Autodesk Inventor part; units mm, degrees
ref_plane "YZ Plane" through (0, 0, 0) normal (1, 0, 0) x (0, 1, 0)
ref_plane "XZ Plane" through (0, 0, 0) normal (0, 1, 0) x (-1, 0, 0)
ref_plane "XY Plane" through (0, 0, 0) normal (0, 0, 1) x (1, 0, 0)
sketch "Sketch1" plane through (0, 0, 0) normal (0, 1, 0) x (-1, 0, 0)
  line L0 (0, 0) -> (50, 0)
  line L1 (50, 0) -> (50, 12.5)
  line L2 (50, 12.5) -> (75, 12.5)
  line L3 (75, 12.5) -> (75, -37.5)
  line L4 (75, -37.5) -> (50, -37.5)
  line L5 (50, -37.5) -> (50, -25)
  line L6 (50, -25) -> (0, -25)
  line L7 (0, -25) -> (0, 0)
  dimension "d0" = 25
  dimension "d1" = 50
  dimension "d2" = 50
  dimension "d3" = 25
extrude "Extrusion1" add sketch "Sketch1" along normal blind 4
sketch "Sketch2" plane through (0, 4, 0) normal (0, 1, 0) x (1, 0, 0)
  circle A0 centre (-15, 12.5) radius 2.75
  circle A1 centre (-35, 12.5) radius 2.75
  circle A2 centre (-62.5, 2.5) radius 2.75
  circle A3 centre (-62.5, 22.5) radius 2.75
  line L0 (-75, -12.5) -> (-50, -12.5)
  line L1 (-62.5, -12.5) -> (-62.5, 37.5) construction
  line L2 (-50, 37.5) -> (-75, 37.5)
  point P0 (0, 0)
  dimension "d6" = 5.5
  dimension "d7" = 5.5
  dimension "d8" = 20
  dimension "d9" = 10
extrude "Extrusion2" cut sketch "Sketch2" against normal through all
fillet "Fillet1" radius 10 2 edges at (-50, 2, 0) (-50, 2, -25)
equation "\"d9\" = 0.5 * d8"
properties part number "Support Extrusion Brace" material "CFRP"
Work out the finished part from the listing and answer in its coordinate system (mm). A direction names the side the tool comes from. Coordinates: 2 decimals unless noted, no trailing zeros. Loops run counter-clockwise (first coordinate to the right, second up) from the corner with the lowest first, then second, coordinate; pieces in that order, holes last. Notation, with made-up numbers: M 86.25,59 L 132.25,59 A12 ccw 132.25,81 Z; hole C 52.25,27 d7. An arc over 180 degrees is marked long. Answer in a Markdown table with one row per item. Add a question column.
1. Find section C-C, the plane x = -62.5. Write down the section's boundary in (y, z).
2. A tool of negligible diameter and unlimited length cuts with its end or side. For faces 1 (the flat face through (-20, 2, 0)), 2 (the flat face through (-20, 2, -25)), 3 (the flat face through (-45, 0, -12)), from which of +Z, -Z, +X, -X, +Y, -Y can it reach the whole face along a straight path? Write none if from no direction.
3. Find section B-B, the plane z = -12.5. Write down the section's boundary in (x, y), then the cut area to 3 significant figures.
4. The mould has two halves that part along Z. Classify faces 4 (the flat face through (-62, 2, 12.5)), 5 (the flat face through (-50, 2, -36)), 6 (the cylindrical face through (-65.247, 2.028, -22.621)): pulls with the +Z half, pulls with the -Z half, needs draft (parallel to the pull), parting line crosses it, or undercut.
5. Flat-ended cylindrical pins translate along their axes: P1, Ø2, axis at y = 2, z = 11.5, coming from the +X side; P2, Ø2, axis at x = -37, y = 1, coming from the +Z side; P3, Ø1, axis at x = -42, y = 1.5, coming from the -Z side; P4, Ø6.5, axis at x = -15, z = -12.5, coming from the +Y side. Find the tip coordinate at first contact, or state that the pin passes through.
6. Find section A-A, the plane x = -35. Write down the section's boundary in (y, z).
7. Find section D-D, the plane y = 3.05. Write down the section's boundary in (x, z).
8. Consider L1, parallel to Z at x = -62.5, y = 2.7; L2, parallel to X at y = 1.2, z = -12.5; L3, parallel to Z at x = -15, y = 2.8. Determine where each line is inside the solid, lowest interval first.
Reported:
| question | item | result |
|---|---|---|
| 1 | outline | M 0,-37.5 L 4,-37.5 L 4,-25.25 L 0,-25.25 Z; M 0,-19.75 L 4,-19.75 L 4,-5.25 L 0,-5.25 Z; M 0,0.25 L 4,0.25 L 4,12.5 L 0,12.5 Z |
| 2 | face 1 | +Z, +X, +Y, -Y |
| 2 | face 2 | -Z, +X, +Y, -Y |
| 2 | face 3 | +Z, -Z, +X, -X, -Y |
| 3 | outline | M -75,0 L -37.75,0 L -37.75,4 L -75,4 Z; M -32.25,0 L -17.75,0 L -17.75,4 L -32.25,4 Z; M -12.25,0 L 0,0 L 0,4 L -12.25,4 Z |
| 3 | area | 256 mm^2 |
| 4 | face 4 | pulls with the +Z half |
| 4 | face 5 | needs draft |
| 4 | face 6 | undercut |
| 5 | P1 | stops at x = -50 |
| 5 | P2 | stops at z = 0 |
| 5 | P3 | stops at z = -25.32 |
| 5 | P4 | stops at y = 4 |
| 6 | outline | M 0,-25 L 4,-25 L 4,-15.25 L 0,-15.25 Z; M 0,-9.75 L 4,-9.75 L 4,0 L 0,0 Z |
| 7 | outline | M -75,-37.5 L -50,-37.5 L -50,-35 A10 cw -40,-25 L 0,-25 L 0,0 L -40,0 A10 cw -50,10 L -50,12.5 L -75,12.5 Z; hole C -62.5,-22.5 d5.5; hole C -62.5,-2.5 d5.5; hole C -35,-12.5 d5.5; hole C -15,-12.5 d5.5 |
| 8 | L1 | z = -37.5 to -25.25, -19.75 to -5.25, 0.25 to 12.5 |
| 8 | L2 | x = -75 to -37.75, -32.25 to -17.75, -12.25 to 0 |
| 8 | L3 | z = -25 to -15.25, -9.75 to 0 |
